Source: three-view drawing plus pictorial views. Frame: mm from the lowest corner of the part. A direction names the side the tool comes from. Give positions to 0.01 mm unless a question says otherwise; leave off trailing zeros. Order: outer loops, then holes, each group sorted by start corner. A loop starts at its lowest first (then second) coordinate and runs counter-clockwise, first axis right, second up. Notation, with made-up numbers: (55, 1) - (93, 1) arc R17 cw to (93, 16) - close; hole circle Ø6 at (9, 25). An arc over 180 degrees is marked (long way). Answer in a Markdown table with one row per item. Add a question column.
1. Section query C-C on y = 16.25. Return loops of the section in (x, z), and give its area (3 significant figures).
2. Access query for the marked faces 4 and 5. Directions: +Z, -Z, +X, -X, +Y, -Y. A direction counts if a zero-diameter tool reaches every point of the face in a straight line with its end or side. Return the directions, or none.
3. Contact query for flat-ended pins moving along their axis: pin 1 (5 mm diameter, centred on x = 60.5, y = 3.5, fed in from +Z); pin 2 (6 mm diameter, centred on y = 16, z = 56, fed in from +X); pin 3 (1 mm diameter, centred on x = 22.5, z = 62.5, fed in from +Y). Output: stop coordinate, or through.
4. Section query A-A on z = 117. Return loops of the section in (x, y), and give its area (3 significant figures).
5. Mould query, pull axis Z, two halves, no side actions, for the marked faces 1, 2 and 3. Classes: released by +Z, released by -Z, zero draft, split by the parting line, or undercut.
6. Section query D-D on x = 18. Return loops of the section in (y, z) (1 decimal), and give its area (3 significant figures).
7. Section query B-B on x = 59.5. Return loops of the section in (y, z) (1 decimal).
8. Ray query, line 1 (X direction, y = 13.75, z = 65); line 2 (Y direction, x = 22.5, z = 91.5). Return the intervals inside material, ascending. Write a range as [from, to].
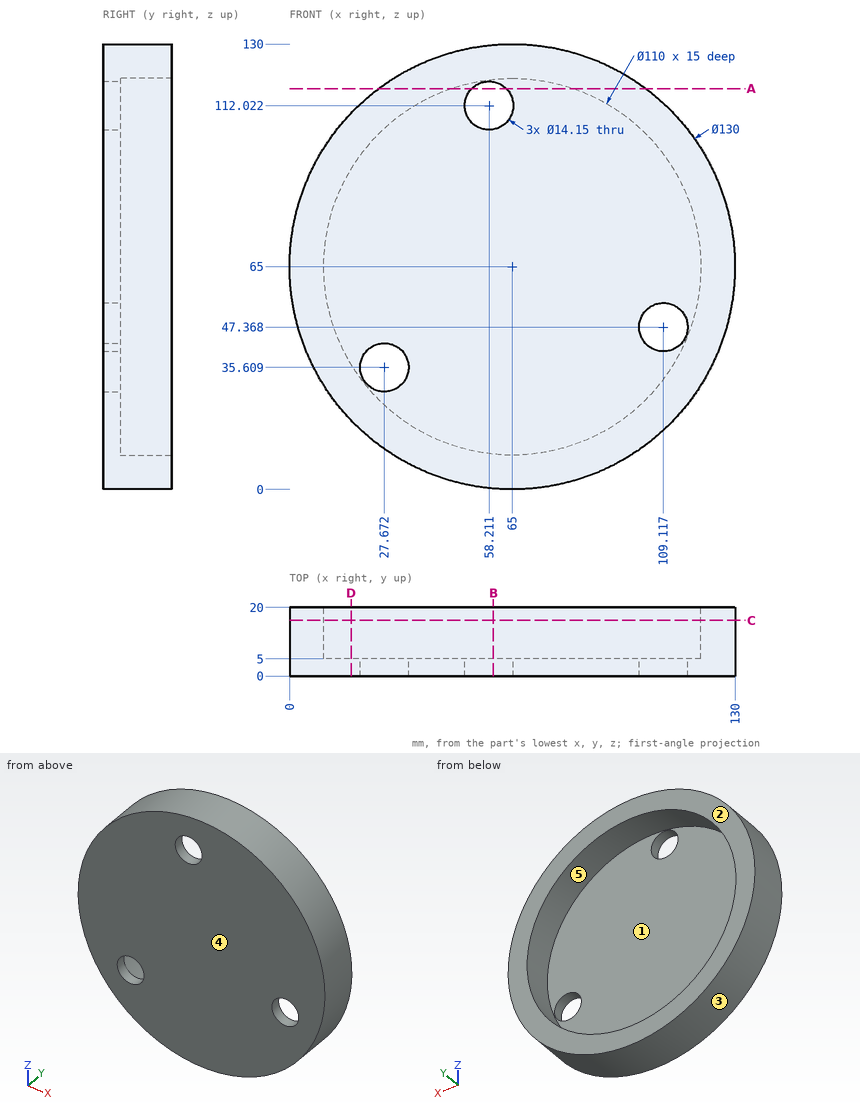
Answer:
| question | item | result |
|---|---|---|
| 1 | outline | circle Ø130 at (65, 65); hole circle Ø110 at (65, 65) |
| 1 | area | 3,770 mm² |
| 2 | face 4 | +Z, -Z, +X, -X, -Y |
| 2 | face 5 | +Y |
| 3 | pin 1 | stops at z = 129.97 |
| 3 | pin 2 | stops at x = 129.72 |
| 3 | pin 3 | stops at y = 5 |
| 4 | outline | (26, 0) - (53.18, 0) - (53.18, 5) - (47.08, 5) - (47.08, 20) - (26, 20) - close; (63.24, 0) - (104, 0) - (104, 20) - (82.92, 20) - (82.92, 5) - (63.24, 5) - close |
| 4 | area | 972 mm² |
| 5 | face 1 | undercut |
| 5 | face 2 | zero draft |
| 5 | face 3 | split by the parting line |
| 6 | outline | (0, 20.1) - (20, 20.1) - (20, 36.4) - (5, 36.4) - (5, 93.6) - (20, 93.6) - (20, 109.9) - (0, 109.9) - close |
| 6 | area | 939 mm² |
| 7 | outline | (0, 0.2) - (20, 0.2) - (20, 10.3) - (5, 10.3) - (5, 105.1) - (0, 105.1) - close; (0, 119) - (5, 119) - (5, 119.7) - (20, 119.7) - (20, 129.8) - (0, 129.8) - close |
| 8 | line 1 | x = [0, 10], [120, 130] |
| 8 | line 2 | y = [0, 5] |
